Could you check a few things on this model? Use its own coordinates, in mm. Face numbers are marked on the shaded views. A direction names the side the tool comes from. Round coordinates to 2 decimals unless told otherwise and drop trailing zeros. Write each loop counter-clockwise with the first axis right and the second up, starting at its lowest first coordinate (ties: lowest second). Pieces come first, ordered by that corner, then holes. Notation, with made-up numbers: (63.5, -12.5) - (119.5, -12.5) arc R5 cw to (119.5, -7.5) - close; hole circle Ø10 at (55.5, 60). An arc over 180 degrees is marked (long way). Write each question's results on one line, items separated by ' | '. Start each with the question number.
(1) Please list where these lines run through material, in increasing order: line 1 (Y direction, x = -2.25, z = 7); line 2 (X direction, y = -18, z = 6.25); line 3 (Y direction, x = -4.75, z = 16). Write a range as [from, to].
(2) Imagine slicing it at A-A on y = -25.5. Write out the boundary of the cut face in (x, z).
(3) Imagine slicing it at C-C on z = 6.25. Write out the boundary of the cut face in (x, y), then the cut area to 3 significant figures.
(4) Imagine slicing it at B-B on x = 4.25. Write out the boundary of the cut face in (y, z), then the cut area to 3 significant figures.
(5) For P1, Ø2.5, axis at x = -1, y = 1, coming from the +Z side; P2, Ø2.5, axis at y = -30.5, z = 1.5, coming from the +X side; P3, Ø5, axis at x = -0.5, y = 13.5, coming from the +Z side; P4, Ø10, axis at y = -19.5, z = 14, coming from the +X side, each with a flat end and sliding along its axis, tell me the tip position at first contact or that it passes through.
(6) Thinking about a two-plate mould opening in Y: for the marked faces 5, 6 and 7, which applies, +Y half, -Y half, draft (parallel to the pull), parting line (faces both ways), or undercut?
(7) Imagine slicing it at D-D on y = 19. Write out the boundary of the cut face in (x, z), then the cut area to 3 significant figures.
(8) On a 3-axis mill with a long thin cutter (end or side, diameter ignored), from which of +Z, -Z, +X, -X, +Y, -Y can I reach the whole of each face in a straight line? I mean the marked faces 1, 2, 3 and 4. Say none if no direction works.
```python
from build123d import *

# Parameters (mm, degrees)
F6_DEPTH       = 10.4
F8_DEPTH       = 22
F9_W           = 15
F9_H           = 3.4
F10_DEPTH      = 24.401
F12_DEPTH      = 10.401
F12_DEPTH_BACK = 10.401
F14_DEPTH      = 8


with BuildPart() as f6:
    # F5 (on Right) → F6 (new body, symmetric)
    with BuildSketch(Plane.YZ):
        with BuildLine():
            Line((24.4, 0), (24.4, 24.4))
            Line((24.4, 24.4), (3.2535533906, 3.2535533906))
            ThreePointArc((3.2535533906, 3.2535533906), (2.7086582838, 3.1451670149), (2.4, 3.6071067812))
            Line((2.4, 3.6071067812), (2.4, 22))
            Line((2.4, 22), (0, 22))
            Line((0, 22), (0, 0))
            Line((0, 0), (24.4, 0))
        make_face()
    extrude(amount=F6_DEPTH, both=True)

    # F7 (on Top) → F8 (join)
    with BuildSketch(Plane.XY):
        with BuildLine():
            Line((-7, 0), (-10.4, 0))
            Line((-10.4, 0), (-10.4, -21.6))
            Line((-10.4, -21.6), (-10.4, -29))
            ThreePointArc((-10.4, -29), (-9.404163056, -31.404163056), (-7, -32.4))
            Line((-7, -32.4), (7, -32.4))
            ThreePointArc((7, -32.4), (9.404163056, -31.404163056), (10.4, -29))
            Line((10.4, -29), (10.4, -21.6))
            Line((10.4, -21.6), (10.4, 0))
            Line((10.4, 0), (7, 0))
            ThreePointArc((7, 0), (7.7071067812, -0.2928932188), (8, -1))
            Line((8, -1), (8, -29))
            ThreePointArc((8, -29), (7.7071067812, -29.7071067812), (7, -30))
            Line((7, -30), (-7, -30))
            ThreePointArc((-7, -30), (-7.7071067812, -29.7071067812), (-8, -29))
            Line((-8, -29), (-8, -1))
            ThreePointArc((-8, -1), (-7.7071067812, -0.2928932188), (-7, 0))
        make_face()
    extrude(amount=F8_DEPTH)

    # F9 (on Top) → F10 (cut, through all)
    with BuildSketch(Plane.XY):
        with Locations((0, -30.7)):
            Rectangle(F9_W, F9_H)
    extrude(amount=F10_DEPTH, mode=Mode.SUBTRACT)

    # F11 (on Right) → F12 (cut, two sides)
    with BuildSketch(Plane.YZ) as f12_sk:
        Polygon((-32.4, 22), (-32.4, 5), (-21.6, 5), (0, 22), align=None)
    extrude(amount=F12_DEPTH, mode=Mode.SUBTRACT)
    extrude(f12_sk.sketch, amount=-F12_DEPTH_BACK, mode=Mode.SUBTRACT)

    # F13 (on Right) → F14 (cut, symmetric)
    with BuildSketch(Plane.YZ):
        Polygon((24.4, 2.4), (24.4, 21.0058874503), (5.7941125497, 2.4), align=None)
    extrude(amount=F14_DEPTH, both=True, mode=Mode.SUBTRACT)


solid = f6.part
```
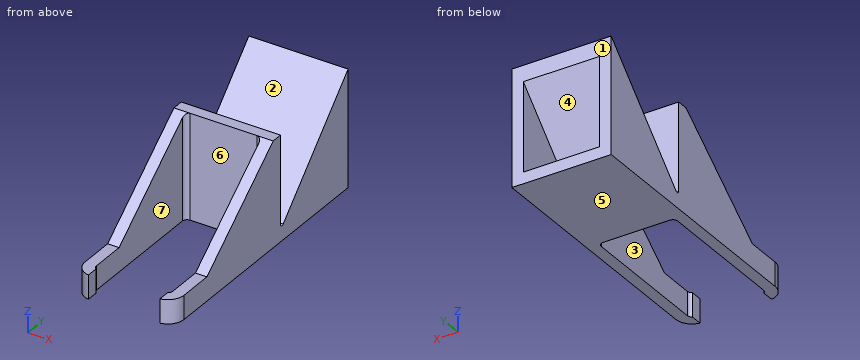
Response:
1) line 1: [0, 2.4], [7, 10.39] | line 2: [-10.4, -8], [8, 10.4] | line 3: [0, 2.4], [16, 19.39]
2) outline: (-10.4, 0) - (-8, 0) - (-8, 5) - (-10.4, 5) - close; (8, 0) - (10.4, 0) - (10.4, 5) - (8, 5) - close
3) outline: (-10.4, -20.01) - (-8, -20.01) - (-8, -1) arc R1 cw to (-7, 0) - (7, 0) arc R1 cw to (8, -1) - (8, -20.01) - (10.4, -20.01) - (10.4, 2.4) - (-10.4, 2.4) - close; (-10.4, 6.25) - (10.4, 6.25) - (10.4, 24.4) - (8, 24.4) - (8, 9.64) - (-8, 9.64) - (-8, 24.4) - (-10.4, 24.4) - close | area: 288 mm²
4) outline: (0, 0) - (24.4, 0) - (24.4, 2.4) - (5.79, 2.4) - (24.4, 21.01) - (24.4, 24.4) - (3.25, 3.25) arc R0.5 cw to (2.4, 3.61) - (2.4, 22) - (0, 22) - close | area: 175 mm²
5) P1: z = 22 | P2: x = 10.39 | P3: z = 16 | P4: through
6) face 5: draft | face 6: -Y half | face 7: undercut
7) outline: (-10.4, 0) - (10.4, 0) - (10.4, 19) - (-10.4, 19) - close; hole (-8, 2.4) - (8, 2.4) - (8, 15.61) - (-8, 15.61) - close | area: 184 mm²
8) face 1: +Z, -Z, +X, -X, +Y | face 2: +Z, +X, -X | face 3: +Z, -Z | face 4: +Y
